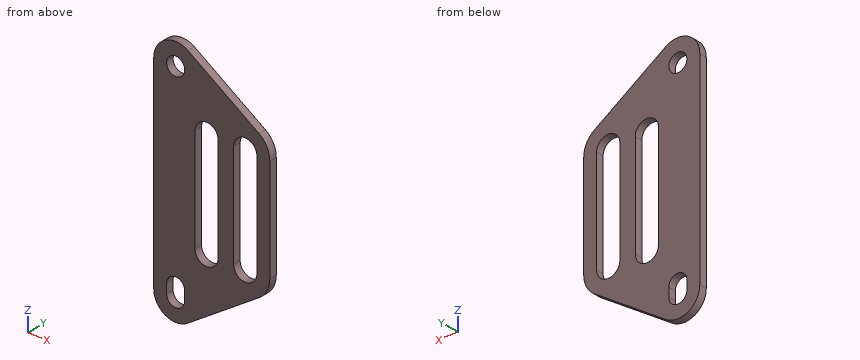
from build123d import *

# Parameters (mm, degrees)
F0_R     = 3.5
F1_DEPTH = 3


with BuildPart() as f1:
    # F0 (on Front) → F1 (new body)
    with BuildSketch(Plane.XZ):
        with BuildLine():
            Line((32.279203, -11.351898), (4.723497, 7.066723))
            ThreePointArc((4.723497, 7.066723), (-4.006262, 7.496657), (-8.5, 0))
            Line((-8.5, 0), (-8.5, -78.5))
            ThreePointArc((-8.5, -78.5), (-4.006262, -85.996657), (4.723497, -85.566723))
            Line((4.723497, -85.566723), (32.279203, -67.148102))
            ThreePointArc((32.279203, -67.148102), (35.378616, -63.727587), (36.5, -59.25))
            Line((36.5, -59.25), (36.5, -19.25))
            ThreePointArc((36.5, -19.25), (35.378616, -14.772413), (32.279203, -11.351898))
        make_face()
        with BuildLine():
            ThreePointArc((-3.5, -75), (0, -71.5), (3.5, -75))
            Line((3.5, -75), (3.5, -78.5))
            ThreePointArc((3.5, -78.5), (0, -82), (-3.5, -78.5))
            Line((-3.5, -78.5), (-3.5, -75))
        make_face(mode=Mode.SUBTRACT)
        with BuildLine():
            ThreePointArc((7.5, -19.25), (12, -14.75), (16.5, -19.25))
            Line((16.5, -19.25), (16.5, -59.25))
            ThreePointArc((16.5, -59.25), (12, -63.75), (7.5, -59.25))
            Line((7.5, -59.25), (7.5, -19.25))
        make_face(mode=Mode.SUBTRACT)
        Circle(F0_R, mode=Mode.SUBTRACT)
        with BuildLine():
            ThreePointArc((22.5, -19.25), (27, -14.75), (31.5, -19.25))
            Line((31.5, -19.25), (31.5, -59.25))
            ThreePointArc((31.5, -59.25), (27, -63.75), (22.5, -59.25))
            Line((22.5, -59.25), (22.5, -19.25))
        make_face(mode=Mode.SUBTRACT)
    extrude(amount=F1_DEPTH)


solid = f1.part
Could you check a few things on this model? Use its own coordinates, in mm. Give positions to 0.01 mm unless a question says otherwise; leave off trailing zeros. Loops run counter-clockwise (first coordinate to the right, second up) from the corner with the lowest first, then second, coordinate; pieces in that order, holes last. Notation, with made-up numbers: M 69.5,2.25 L 75.5,2.25 A30 ccw 75.5,34.25 Z; hole C 23,33 d1. An arc over 180 degrees is marked long. Answer as a JSON object with one key per item and string values.
Q1. For P1, Ø1.5, axis at y = -1, z = -77.5, coming from the +X side; P2, Ø1.5, axis at x = 14, z = -38, coming from the +Y side, each with a flat end and sliding along its axis, tell me the tip position at first contact or that it passes through.
Values found:
{"P1": "stops at x = 17.91", "P2": "passes through"}
Q2. If I drill on probe 1 along X at (y, z) = (-1.6, -45.5); probe 2 along Z at (x, y) = (0, -1.6); probe 3 along X at (y, z) = (-2.3, -18), over which ranges is the centre line in solid material (lowest first)? Write a range as [from, to].
Values found:
{"probe 1": "x = [-8.5, 7.5], [16.5, 22.5], [31.5, 36.5]", "probe 2": "z = [-87, -82], [-71.5, -3.5], [3.5, 8.5]", "probe 3": "x = [-8.5, 7.68], [16.32, 22.68], [31.32, 36.42]"}
Q3. Suppose I cut it at D-D, the plane x = 27. List the corners of the cut face in (y, z) for me, plus the area to 3 significant figures.
Values found:
{"outline": "M -3,-70.68 L 0,-70.68 L 0,-63.75 L -3,-63.75 Z; M -3,-14.75 L 0,-14.75 L 0,-7.82 L -3,-7.82 Z", "area": "41.6 mm²"}
Q4. Suppose I cut it at C-C, the plane x = 2. List the corners of the cut face in (y, z) for me.
Values found:
{"outline": "M -3,-86.76 L 0,-86.76 L 0,-81.37 L -3,-81.37 Z; M -3,-72.13 L 0,-72.13 L 0,-2.87 L -3,-2.87 Z; M -3,2.87 L 0,2.87 L 0,8.26 L -3,8.26 Z"}
Q5. Suppose I cut it at B-B, the plane y = -1.65. List the corners of the cut face in (x, z) for me.
Values found:
{"outline": "M -8.5,-78.5 A8.5 ccw 4.72,-85.57 L 32.28,-67.15 A9.5 ccw 36.5,-59.25 L 36.5,-19.25 A9.5 ccw 32.28,-11.35 L 4.72,7.07 A8.5 ccw -8.5,0 Z; hole M -3.5,-78.5 A3.5 ccw 3.5,-78.5 L 3.5,-75 A3.5 ccw -3.5,-75 Z; hole C 0,0 d7; hole M 7.5,-59.25 A4.5 ccw 16.5,-59.25 L 16.5,-19.25 A4.5 ccw 7.5,-19.25 Z; hole M 22.5,-59.25 A4.5 ccw 31.5,-59.25 L 31.5,-19.25 A4.5 ccw 22.5,-19.25 Z"}
Q6. Suppose I cut it at A-A, the plane z = -50. List the corners of the cut face in (x, y) for me, plus the area to 3 significant figures.
Values found:
{"outline": "M -8.5,-3 L 7.5,-3 L 7.5,0 L -8.5,0 Z; M 16.5,-3 L 22.5,-3 L 22.5,0 L 16.5,0 Z; M 31.5,-3 L 36.5,-3 L 36.5,0 L 31.5,0 Z", "area": "81.0 mm²"}
